```python
from build123d import *

# Parameters (mm, degrees)
SKETCH1_R                = 3.75
BOSS_EXTRUDE1_DEPTH      = 12
SKETCH1_3_R              = 3.75
BOSS_EXTRUDE2_DEPTH      = 16
BOSS_EXTRUDE2_DEPTH_BACK = 4
BOSS_EXTRUDE3_DEPTH      = 16


with BuildPart() as part:
    # Sketch1 → Boss-Extrude1 (new body)
    with BuildSketch(Plane(origin=(0, 0, 0), x_dir=(1, 0, 0), z_dir=(0, 1, 0))):
        with BuildLine():
            Line((82, 8), (-82, 8))
            ThreePointArc((-82, 8), (-76.343145751, 5.656854249), (-74, 0))
            ThreePointArc((-74, 0), (-76.343145751, -5.656854249), (-82, -8))
            Line((-82, -8), (82, -8))
            ThreePointArc((82, -8), (74, 0), (82, 8))
        make_face()
        with BuildLine():
            ThreePointArc((-74, 0), (-76.343145751, 5.656854249), (-82, 8))
            ThreePointArc((-82, 8), (-90, 0), (-82, -8))
            ThreePointArc((-82, -8), (-76.343145751, -5.656854249), (-74, 0))
        make_face()
        with Locations((-82, 0)):
            Circle(SKETCH1_R, mode=Mode.SUBTRACT)
        with BuildLine():
            ThreePointArc((90, 0), (87.656854249, 5.656854249), (82, 8))
            ThreePointArc((82, 8), (74, 0), (82, -8))
            ThreePointArc((82, -8), (87.656854249, -5.656854249), (90, 0))
        make_face()
        with Locations((82, 0)):
            Circle(SKETCH1_R, mode=Mode.SUBTRACT)
    extrude(amount=BOSS_EXTRUDE1_DEPTH)

    # Sketch1_3 → Boss-Extrude2 (add, two sides)
    with BuildSketch(Plane(origin=(0, 0, 0), x_dir=(1, 0, 0), z_dir=(0, 1, 0))) as boss_extrude2_sk:
        with BuildLine():
            ThreePointArc((-74, 0), (-76.343145751, 5.656854249), (-82, 8))
            ThreePointArc((-82, 8), (-90, 0), (-82, -8))
            ThreePointArc((-82, -8), (-76.343145751, -5.656854249), (-74, 0))
        make_face()
        with Locations((-82, 0)):
            Circle(SKETCH1_3_R, mode=Mode.SUBTRACT)
        with BuildLine():
            ThreePointArc((90, 0), (87.656854249, 5.656854249), (82, 8))
            ThreePointArc((82, 8), (74, 0), (82, -8))
            ThreePointArc((82, -8), (87.656854249, -5.656854249), (90, 0))
        make_face()
        with Locations((82, 0)):
            Circle(SKETCH1_3_R, mode=Mode.SUBTRACT)
    extrude(amount=BOSS_EXTRUDE2_DEPTH)
    extrude(boss_extrude2_sk.sketch, amount=-BOSS_EXTRUDE2_DEPTH_BACK)

    # Sketch2 → Boss-Extrude3 (add)
    with BuildSketch(Plane.XY.offset(8)):
        Polygon((-72, 12), (-71.090074414, 14.5), (-69.090074414, 14.5), (-68.180148829, 12), align=None)
        Polygon((-62.180148829, 12), (-66, 12), (-65.090074414, 14.5), (-63.090074414, 14.5), align=None)
        Polygon((-56.180148829, 12), (-60, 12), (-59.090074414, 14.5), (-57.090074414, 14.5), align=None)
        Polygon((-50.180148829, 12), (-54, 12), (-53.090074414, 14.5), (-51.090074414, 14.5), align=None)
        Polygon((-44.180148829, 12), (-48, 12), (-47.090074414, 14.5), (-45.090074414, 14.5), align=None)
        Polygon((-38.180148829, 12), (-42, 12), (-41.090074414, 14.5), (-39.090074414, 14.5), align=None)
        Polygon((-32.180148829, 12), (-36, 12), (-35.090074414, 14.5), (-33.090074414, 14.5), align=None)
        Polygon((-26.180148829, 12), (-30, 12), (-29.090074414, 14.5), (-27.090074414, 14.5), align=None)
        Polygon((-20.180148829, 12), (-24, 12), (-23.090074414, 14.5), (-21.090074414, 14.5), align=None)
        Polygon((-14.180148829, 12), (-18, 12), (-17.090074414, 14.5), (-15.090074414, 14.5), align=None)
        Polygon((-8.180148829, 12), (-12, 12), (-11.090074414, 14.5), (-9.090074414, 14.5), align=None)
        Polygon((-2.180148829, 12), (-6, 12), (-5.090074414, 14.5), (-3.090074414, 14.5), align=None)
        Polygon((3.819851171, 12), (0, 12), (0.909925586, 14.5), (2.909925586, 14.5), align=None)
        Polygon((9.819851171, 12), (6, 12), (6.909925586, 14.5), (8.909925586, 14.5), align=None)
        Polygon((15.819851171, 12), (12, 12), (12.909925586, 14.5), (14.909925586, 14.5), align=None)
        Polygon((21.819851171, 12), (18, 12), (18.909925586, 14.5), (20.909925586, 14.5), align=None)
        Polygon((27.819851171, 12), (24, 12), (24.909925586, 14.5), (26.909925586, 14.5), align=None)
        Polygon((33.819851171, 12), (30, 12), (30.909925586, 14.5), (32.909925586, 14.5), align=None)
        Polygon((39.819851171, 12), (36, 12), (36.909925586, 14.5), (38.909925586, 14.5), align=None)
        Polygon((45.819851171, 12), (42, 12), (42.909925586, 14.5), (44.909925586, 14.5), align=None)
        Polygon((51.819851171, 12), (48, 12), (48.909925586, 14.5), (50.909925586, 14.5), align=None)
        Polygon((57.819851171, 12), (54, 12), (54.909925586, 14.5), (56.909925586, 14.5), align=None)
        Polygon((63.819851171, 12), (60, 12), (60.909925586, 14.5), (62.909925586, 14.5), align=None)
        Polygon((69.819851171, 12), (66, 12), (66.909925586, 14.5), (68.909925586, 14.5), align=None)
    extrude(amount=-BOSS_EXTRUDE3_DEPTH)


solid = part.part
```
For this review, take the finished solid that the model builds, in its own axes (mm). A direction names the side the tool comes from. Coordinates: 2 decimals unless noted, no trailing zeros. Write each loop counter-clockwise with the first axis right and the second up, starting at its lowest first coordinate (ties: lowest second). Pieces come first, ordered by that corner, then holes.
(1) Tool access review of faces 4 (the face through (73, 12, 0)), 5 (the face through (-78.56, -4, -1.89)): name each direction out of +Z, -Z, +X, -X, +Y, -Y from which nothing blocks a thin tool from reaching the whole face with its end or side.
(2) For pin 1 Ø3 at (x, z) = (-52.5, -1) entering from -Y; pin 2 Ø2 at (x, z) = (19.5, -2.5) entering from +Y; pin 3 Ø5 at (y, z) = (13.5, 3.5) entering from +X, all flat-tipped, find the tip position at first contact; note any pin that passes through.
(3) Add section B-B on z = 2. Count the separate pieces of the cut face and the enclosed holes in it, then the cut area to 3 significant figures.
(4) The part is to be moulded in two halves that separate along X. For faces 1 (the face through (85.44, -4, -1.89)), 2 (the face through (-73.7, 12, 0)), 3 (the face through (-1, 0, 0)), say which applies: +X half, -X half, draft (parallel to the pull), parting line (faces both ways), or undercut.
(5) Add section A-A on y = -2.25. Give the boundary of the cut face in (x, z), then the cut area to 3 significant figures.
(6) Wall thickness on probe 1 along X at (y, z) = (0.25, -2.5); probe 2 along X at (y, z) = (-0.25, 1.5); probe 3 along Z at (x, y) = (-82, 6.5): over which ranges is each line inside the solid? List them lowest first.
Answer sheet:
1. face 4: +Y
1. face 5: +Z, -Z, +X, -X, -Y
2. pin 1: stops at y = 0
2. pin 2: stops at y = 14.5
2. pin 3: stops at x = 89.94
3. separate pieces: 3
3. enclosed holes: 0
3. area: 2,320 mm2
4. face 1: draft
4. face 2: undercut
4. face 3: undercut
5. outline: circle Ø16 at (-82, 0); circle Ø16 at (82, 0); hole circle Ø7.5 at (-82, 0); hole circle Ø7.5 at (82, 0)
5. area: 314 mm2
6. probe 1: x = -89.6 to -84.8, -79.2 to 79.2, 84.8 to 89.6
6. probe 2: x = -89.86 to -85.44, -78.56 to -74.14, 74.14 to 78.56, 85.44 to 89.86
6. probe 3: z = -8 to -3.75, 3.75 to 8
